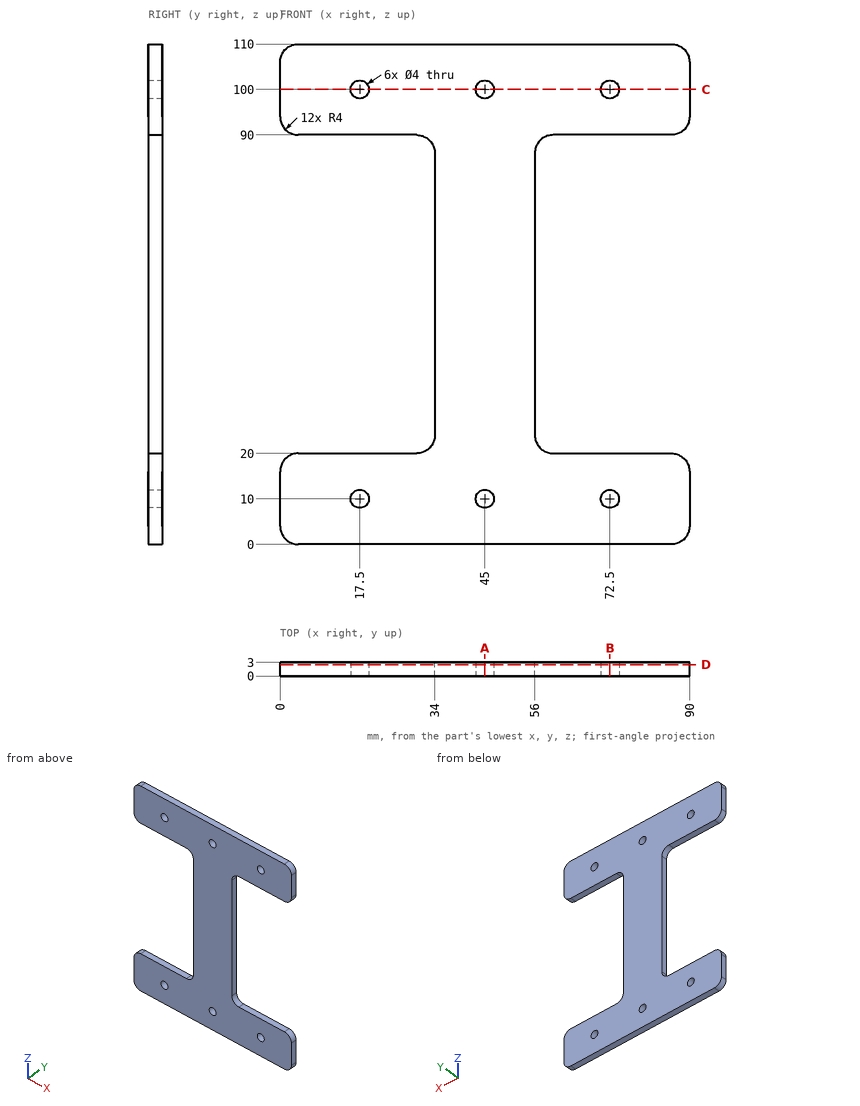
Geometry check sheet. Reference: drawing and pictorial views, mm from the part's lowest x, y, z. Round coordinates to 2 decimals unless told otherwise and drop trailing zeros. Order: outer loops, then holes, each group sorted by start corner. A loop starts at its lowest first (then second) coordinate and runs counter-clockwise, first axis right, second up. Notation, with made-up numbers: (-11.5, -5.5) -> (29.5, -5.5) arc R23 ccw to (29.5, 32.5) -> close; hole circle Ø9 at (76.5, 45.25). An arc over 180 degrees is marked (long way). One line per item, written item: value. Start each with the question number.
Q1. Cross-section at C-C (z = 100). Record the boundary of the cut face in (x, y).
Q2. Thickness scan on line 1 (X direction, y = 0.9, z = 100); line 2 (Z direction, x = 72.5, y = 2); line 3 (Z direction, x = 81, y = 2.25). Record the ranges inside material, lowest first.
Q3. Gauge pin test, flat ends, axial feed: pin 1 Ø1.5 at (y, z) = (1.5, 59) entering from -X; pin 2 Ø0.9 at (y, z) = (1, 69) entering from +X. Record the tip position at first contact, or that the pin passes through.
Q4. Cross-section at D-D (y = 2.5). Give the number of separate pieces and of enclosed holes in the cut face, and give its area (3 significant figures).
Q5. Cross-section at B-B (x = 72.5). Record the boundary of the cut face in (y, z).
Q6. Cross-section at A-A (x = 45). Record the boundary of the cut face in (y, z).
Completed:
1. outline: (0, 0) -> (15.5, 0) -> (15.5, 3) -> (0, 3) -> close; (19.5, 0) -> (43, 0) -> (43, 3) -> (19.5, 3) -> close; (47, 0) -> (70.5, 0) -> (70.5, 3) -> (47, 3) -> close; (74.5, 0) -> (90, 0) -> (90, 3) -> (74.5, 3) -> close
2. line 1: x = 0 to 15.5, 19.5 to 43, 47 to 70.5, 74.5 to 90
2. line 2: z = 0 to 8, 12 to 20, 90 to 98, 102 to 110
2. line 3: z = 0 to 20, 90 to 110
3. pin 1: stops at x = 34
3. pin 2: stops at x = 56
4. separate pieces: 1
4. enclosed holes: 6
4. area: 5,050 mm²
5. outline: (0, 0) -> (3, 0) -> (3, 8) -> (0, 8) -> close; (0, 12) -> (3, 12) -> (3, 20) -> (0, 20) -> close; (0, 90) -> (3, 90) -> (3, 98) -> (0, 98) -> close; (0, 102) -> (3, 102) -> (3, 110) -> (0, 110) -> close
6. outline: (0, 0) -> (3, 0) -> (3, 8) -> (0, 8) -> close; (0, 12) -> (3, 12) -> (3, 98) -> (0, 98) -> close; (0, 102) -> (3, 102) -> (3, 110) -> (0, 110) -> close
